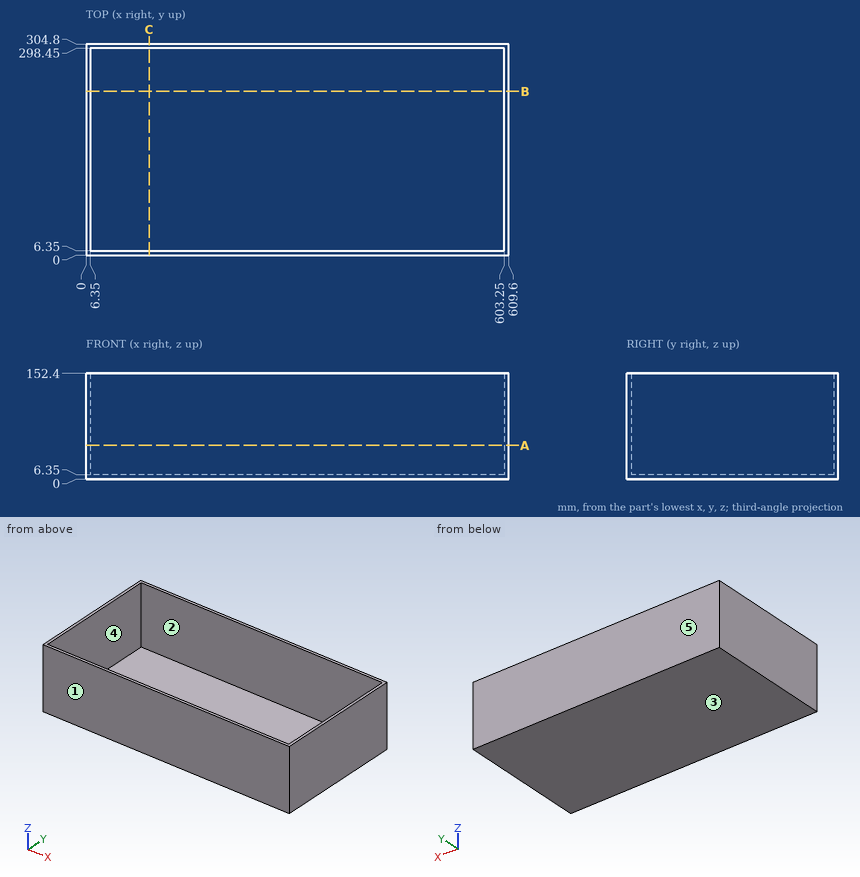
Design review of the part shown in the three views and the two pictorial views. Dimensions are in mm from the part's minimum x, y and z. A direction names the side the tool comes from. Coordinates: 2 decimals unless noted, no trailing zeros. Write each loop counter-clockwise with the first axis right and the second up, starting at its lowest first coordinate (ties: lowest second). Pieces come first, ordered by that corner, then holes. Notation, with made-up numbers: (49, 38) -> (85, 38) arc R11 ccw to (85, 59) -> close; hole circle Ø9 at (-38.5, 6.5). An arc over 180 degrees is marked (long way). Answer in a Markdown table with one row per item.
1. Wall thickness on probe 1 along X at (y, z) = (254, 61.5); probe 2 along Y at (x, z) = (311.5, 145.5); probe 3 along Z at (x, y) = (395, 224.5): over which ranges is each line inside the solid? List them lowest first. Write a range as [from, to].
Answers below:
| item | result |
|---|---|
| probe 1 | x = [0, 6.35], [603.25, 609.6] |
| probe 2 | y = [0, 6.35], [298.45, 304.8] |
| probe 3 | z = [0, 6.35] |
2. We need section B-B, the plane y = 236.5. State the section outline as (x, z) points, and give its area (3 significant figures).
Answers below:
| item | result |
|---|---|
| outline | (0, 0) -> (609.6, 0) -> (609.6, 152.4) -> (603.25, 152.4) -> (603.25, 6.35) -> (6.35, 6.35) -> (6.35, 152.4) -> (0, 152.4) -> close |
| area | 5,730 mm^2 |
3. Draft analysis for pull direction Y (two halves, no side actions). For the marked faces 3, 4 and 5, state which applies: +Y half, -Y half, draft (parallel to the pull), parting line (faces both ways), or undercut.
Answers below:
| item | result |
|---|---|
| face 3 | draft |
| face 4 | undercut |
| face 5 | +Y half |
4. We need section C-C, the plane x = 91. State the section outline as (y, z) points, and give its area (3 significant figures).
Answers below:
| item | result |
|---|---|
| outline | (0, 0) -> (304.8, 0) -> (304.8, 152.4) -> (298.45, 152.4) -> (298.45, 6.35) -> (6.35, 6.35) -> (6.35, 152.4) -> (0, 152.4) -> close |
| area | 3,790 mm^2 |
5. For the marked faces 1 and 2, list the 3-axis set-ups (+Z, -Z, +X, -X, +Y, -Y) from which the entire face can be reached by the end or side of a thin tool; tool diameter is ignored.
Answers below:
| item | result |
|---|---|
| face 1 | +Z, -Z, +X, -X, -Y |
| face 2 | +Z |
6. We need section A-A, the plane z = 48.5. State the section outline as (x, y) points, and give its area (3 significant figures).
Answers below:
| item | result |
|---|---|
| outline | (0, 0) -> (609.6, 0) -> (609.6, 304.8) -> (0, 304.8) -> close; hole (6.35, 6.35) -> (603.25, 6.35) -> (603.25, 298.45) -> (6.35, 298.45) -> close |
| area | 11,500 mm^2 |
7. Clearance check with flat-ended pins moving along their axes: pin 1 Ø10 at (x, y) = (134, 145) entering from +Z; pin 2 Ø10 at (x, y) = (185.5, 180) entering from -Z. State where each tip first meets the part, or that it passes through.
Answers below:
| item | result |
|---|---|
| pin 1 | stops at z = 6.35 |
| pin 2 | stops at z = 0 |
